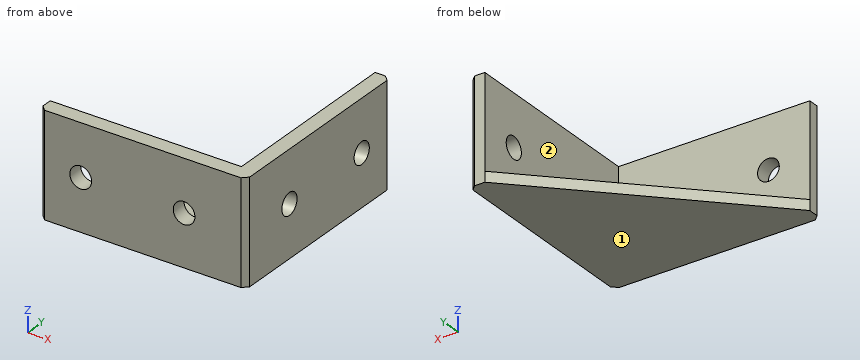
from build123d import *

# Parameters (mm, degrees)
ESQUISSE1_W             = 40
ESQUISSE1_H             = 40
BOSS_EXTRU_1_DEPTH      = 20
ESQUISSE2_W             = 37
ESQUISSE2_H             = 37
ENL_V_MAT_EXTRU_1_DEPTH = 18
ENL_V_MAT_EXTRU_2_DEPTH = 3
CHANFREIN1_SIZE         = 1
ESQUISSE4_R             = 2.1
ENL_V_MAT_EXTRU_3_DEPTH = 4
ESQUISSE5_R             = 2.1
ENL_V_MAT_EXTRU_4_DEPTH = 4


with BuildPart() as part:
    # Esquisse1 → Boss.-Extru.1 (new body)
    with BuildSketch(Plane.XY):
        with Locations((-20, 20)):
            Rectangle(ESQUISSE1_W, ESQUISSE1_H)
    extrude(amount=BOSS_EXTRU_1_DEPTH)

    # Esquisse2 → Enlèv. mat.-Extru.1 (cut)
    with BuildSketch(Plane.XY.offset(20)):
        with Locations((-21.5, 21.5)):
            Rectangle(ESQUISSE2_W, ESQUISSE2_H)
    extrude(amount=-ENL_V_MAT_EXTRU_1_DEPTH, mode=Mode.SUBTRACT)

    # Esquisse3 → Enlèv. mat.-Extru.2 (cut, through all)
    with BuildSketch(Plane.XY.offset(2)):
        Polygon((-40, 3), (-3, 40), (-40, 40), align=None)
    extrude(amount=-ENL_V_MAT_EXTRU_2_DEPTH, mode=Mode.SUBTRACT)

    # Chanfrein1
    chanfrein1_edges = [part.edges().sort_by_distance(p)[0] for p in [
        (0, 0, 10),
        (-40, 0, 10),
        (0, 40, 10),
    ]]
    chamfer(chanfrein1_edges, length=CHANFREIN1_SIZE)

    # Esquisse4 → Enlèv. mat.-Extru.3 (cut, through all)
    with BuildSketch(Plane(origin=(0, 3, 0), x_dir=(1, 0, 0), z_dir=(0, 1, 0))):
        with Locations((-12, -10)):
            Circle(ESQUISSE4_R)
        with Locations((-32, -10)):
            Circle(ESQUISSE4_R)
    extrude(amount=-ENL_V_MAT_EXTRU_3_DEPTH, mode=Mode.SUBTRACT)

    # Esquisse5 → Enlèv. mat.-Extru.4 (cut, through all)
    with BuildSketch(Plane.ZY.offset(3)):
        with Locations((10, 12)):
            Circle(ESQUISSE5_R)
        with Locations((10, 32)):
            Circle(ESQUISSE5_R)
    extrude(amount=-ENL_V_MAT_EXTRU_4_DEPTH, mode=Mode.SUBTRACT)


solid = part.part
Check sheet for the modelled part. Datum: model origin and axes. Units: mm. Face numbers are marked on the shaded views. A direction names the side the tool comes from. Round coordinates to 2 decimals unless told otherwise and drop trailing zeros. Loops run counter-clockwise (first coordinate to the right, second up) from the corner with the lowest first, then second, coordinate; pieces in that order, holes last. Notation, with made-up numbers: (37, 85.25) -> (46, 85.25) arc R29 ccw to (46, 119.25) -> close; hole circle Ø1 at (85.25, 29). An arc over 180 degrees is marked (long way). Put each result on its own line as item: value. Start each with the question number.
1. Section check B-B (z = 10). Enter the section's corners in (x, y), plus the area to 3 significant figures.
2. Scan lines: probe 1 along Y at (x, z) = (-2, 10); probe 2 along X at (y, z) = (1.5, 10); probe 3 along Y at (x, z) = (-20.5, 7.5). Record each from-to range of solid material in increasing order.
3. Gauge pin test, flat ends, axial feed: pin 1 (18.5 mm diameter, centred on x = -23.5, y = 16, fed in from +Z); pin 2 (3 mm diameter, centred on x = -31.5, z = 11, fed in from +Y); pin 3 (12 mm diameter, centred on y = 24, z = 11.5, fed in from -X). Record the tip position at first contact, or that the pin passes through.
4. Section check C-C (y = 12). Enter the section's corners in (x, z), plus the area to 3 significant figures.
5. Access from +Z, -Z, +X, -X, +Y, -Y to the whole of each face (thin tool, end or side, straight path). Record for the marked faces 1 and 2.
6. Section check D-D (z = 7). Enter the section's corners in (x, y).
7. Section check A-A (x = -12). Enter the section's corners in (y, z).
Findings:
1. outline: (-40, 1) -> (-39, 0) -> (-34.1, 0) -> (-34.1, 3) -> (-40, 3) -> close; (-29.9, 0) -> (-14.1, 0) -> (-14.1, 3) -> (-29.9, 3) -> close; (-9.9, 0) -> (-1, 0) -> (0, 1) -> (0, 9.9) -> (-3, 9.9) -> (-3, 3) -> (-9.9, 3) -> close; (-3, 14.1) -> (0, 14.1) -> (0, 29.9) -> (-3, 29.9) -> close; (-3, 34.1) -> (0, 34.1) -> (0, 39) -> (-1, 40) -> (-3, 40) -> close
1. area: 179 mm^2
2. probe 1: y = 0 to 9.9, 14.1 to 29.9, 34.1 to 40
2. probe 2: x = -40 to -34.1, -29.9 to -14.1, -9.9 to 0
2. probe 3: y = 0 to 3
3. pin 1: stops at z = 2
3. pin 2: stops at y = 3
3. pin 3: stops at x = -3
4. outline: (-31, 0) -> (0, 0) -> (0, 7.9) -> (-3, 7.9) -> (-3, 2) -> (-31, 2) -> close; (-3, 12.1) -> (0, 12.1) -> (0, 20) -> (-3, 20) -> close
4. area: 103 mm^2
5. face 1: -Z, +X, -X, +Y, -Y
5. face 2: +Z, -X, +Y
6. outline: (-40, 1) -> (-39, 0) -> (-1, 0) -> (0, 1) -> (0, 39) -> (-1, 40) -> (-3, 40) -> (-3, 3) -> (-40, 3) -> close
7. outline: (0, 0) -> (31, 0) -> (31, 2) -> (3, 2) -> (3, 7.9) -> (0, 7.9) -> close; (0, 12.1) -> (3, 12.1) -> (3, 20) -> (0, 20) -> close
